Input: part model. Units: mm. Frame: model coordinates. Face numbers are marked on the shaded views. A direction names the side the tool comes from. Round coordinates to 2 decimals unless told otherwise and drop trailing zeros. Write each loop counter-clockwise with the first axis right and the second up, starting at its lowest first coordinate (ties: lowest second). Pieces come first, ordered by that corner, then holes. Notation, with made-up numbers: M 73,84 L 106,84 A4 ccw 106,89 Z; hole C -27.5,-4 d6. An arc over 180 degrees is marked long. Use one line per item in the form item = value. Start each with the question number.
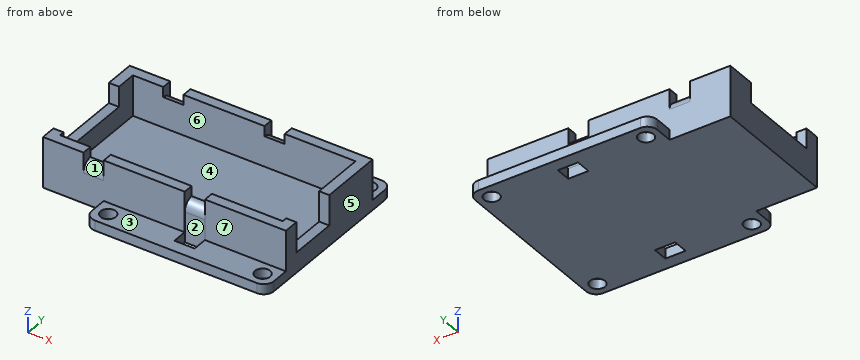
```python
from build123d import *

# Parameters (mm, degrees)
F1_DEPTH     = 2
F2_R         = 2
F3_D         = 3
F6_W         = 2
F6_H         = 9.5
F7_DEPTH     = 2
F6_W_2       = 4
F6_H_2       = 2
F6_H_3       = 1.9668334348
F8_DEPTH     = 8
F6_W_3       = 16
F9_DEPTH     = 10
F10_T1_DEPTH = 4
F10_T3_DEPTH = 4
F11_DEPTH    = 4
F6_H_4       = 16
F12_DEPTH    = 6


# Not quite as in the source:
# - a fillet or chamfer that OpenCascade refuses, or shapes differently, is made with other operations: its cross-section is extruded or revolved along the edge and cut away or added
# - a feature names something its author has since deleted; it is built from what else it names


with BuildPart() as f1:
    # F0 (on Top) → F1 (new body)
    with BuildSketch(Plane.XY):
        Polygon((-19.8978664808, -19.9668334348), (-1.8978664808, -19.9668334348), (-1.8978664808, -17.4668334348), (-3.8978664808, -17.4668334348), (-3.8978664808, -14.4668334348), (-1.8978664808, -14.4668334348), (-1.8978664808, -1.9668334348), (-19.8978664808, -1.9668334348), align=None)
    extrude(amount=F1_DEPTH)

    # F2
    f2_edges = [f1.edges().sort_by_distance(p)[0] for p in [
        (-19.897866, -19.966833, 1),
    ]]
    fillet(f2_edges, radius=F2_R)

    # F3 (through all)
    with Locations(Plane(origin=(0, 0, 0), x_dir=(1, 0, 0), z_dir=(0, 0, -1))):
        with Locations((-17.1478664808, 17.2168334348)):
            Hole(F3_D / 2)

    # F4: F1 across face


with BuildPart() as f1_1:
    add(f1.part)
    add(f1.part.mirror(Plane(origin=(-1.8978664808, -8.2168334348, 1), x_dir=(0, 1, 0), z_dir=(1, 0, 0))))

    # F5: F1 across face


with BuildPart() as f1_2:
    add(f1_1.part)
    add(f1_1.part.mirror(Plane(origin=(-1.8978664808, -1.9668334348, 1), x_dir=(-1, 0, 0), z_dir=(0, 1, 0))))

    # F6 (on face) → F7 (join)
    with BuildSketch(Plane(origin=(0, 0, 0), x_dir=(1, 0, 0), z_dir=(0, 0, -1))):
        Polygon((-29.8978664808, -8.5), (-23.8978664808, -8.5), (-19.8978664808, -8.5), (-19.8978664808, 12.5), (-23.8978664808, 12.5), (-29.8978664808, 12.5), (-29.8978664808, 11.5), (-29.8978664808, -4.5), align=None)
        with Locations((15.1021335192, 6.75)):
            Rectangle(F6_W, F6_H)
        Polygon((-19.8978664808, 12.5), (-19.8978664808, -8.5), (-3.8978664808, -8.5), (0.1021335192, -8.5), (14.1021335192, -8.5), (14.1021335192, 2), (14.1021335192, 11.5), (14.1021335192, 12.5), (0.1021335192, 12.5), (-3.8978664808, 12.5), align=None)
    extrude(amount=-F7_DEPTH)

    # F6 (on face) → F8 (join)
    with BuildSketch(Plane(origin=(0, 0, 0), x_dir=(1, 0, 0), z_dir=(0, 0, -1))):
        with Locations((-1.8978664808, -9.5)):
            Rectangle(F6_W_2, F6_H_2)
        with Locations((-1.8978664808, 13.4834167174)):
            Rectangle(F6_W_2, F6_H_3)
        with Locations((-21.8978664808, 13.5)):
            Rectangle(F6_W_2, F6_H_2)
        with Locations((-21.8978664808, -9.5)):
            Rectangle(F6_W_2, F6_H_2)
    extrude(amount=-F8_DEPTH)

    # F6 (on face) → F9 (join)
    with BuildSketch(Plane(origin=(0, 0, 0), x_dir=(1, 0, 0), z_dir=(0, 0, -1))):
        Polygon((-31.8978664808, -10.5), (-23.8978664808, -10.5), (-23.8978664808, -8.5), (-29.8978664808, -8.5), (-29.8978664808, -4.5), (-31.8978664808, -4.5), align=None)
        Polygon((0.1021335192, -8.5), (0.1021335192, -10.5), (16.1021335192, -10.5), (16.1021335192, 2), (14.1021335192, 2), (14.1021335192, -8.5), align=None)
        Polygon((0.1021335192, 14.4668334348), (0.1021335192, 12.5), (14.1021335192, 12.5), (14.1021335192, 11.5), (16.1021335192, 11.5), (16.1021335192, 14.5), (0.1021335192, 14.5), align=None)
        Polygon((-19.8978664808, 14.5), (-19.8978664808, 12.5), (-3.8978664808, 12.5), (-3.8978664808, 14.4668334348), (-3.8978664808, 14.5), align=None)
        Polygon((-31.8978664808, 14.5), (-31.8978664808, 11.5), (-29.8978664808, 11.5), (-29.8978664808, 12.5), (-23.8978664808, 12.5), (-23.8978664808, 14.5), align=None)
        with Locations((-11.8978664808, -9.5)):
            Rectangle(F6_W_3, F6_H_2)
    extrude(amount=-F9_DEPTH)

    # F10: fillet of radius 2 on 4 edges, made by hand

    # F10_s2 → F10_t1 (cut)
    with BuildSketch(Plane.YZ.offset(-3.8978664808)):
        with BuildLine():
            ThreePointArc((-14.4668334348, 6), (-13.8810469972, 7.4142135624), (-12.4668334348, 8))
            Line((-12.4668334348, 8), (-14.4668334348, 8))
            Line((-14.4668334348, 8), (-14.4668334348, 6))
        make_face()
        with BuildLine():
            ThreePointArc((8.5, 8), (9.9142135624, 7.4142135624), (10.5, 6))
            Line((10.5, 6), (10.5, 8))
            Line((10.5, 8), (8.5, 8))
        make_face()
    extrude(amount=F10_T1_DEPTH, mode=Mode.SUBTRACT)

    # F10_s4 → F10_t3 (cut)
    with BuildSketch(Plane.YZ.offset(-23.8978664808)):
        with BuildLine():
            ThreePointArc((8.5, 8), (9.9142135624, 7.4142135624), (10.5, 6))
            Line((10.5, 6), (10.5, 8))
            Line((10.5, 8), (8.5, 8))
        make_face()
        with BuildLine():
            ThreePointArc((-14.5, 6), (-13.9142135624, 7.4142135624), (-12.5, 8))
            Line((-12.5, 8), (-14.5, 8))
            Line((-14.5, 8), (-14.5, 6))
        make_face()
    extrude(amount=F10_T3_DEPTH, mode=Mode.SUBTRACT)

    # F6 (on face) → F11 (join)
    with BuildSketch(Plane(origin=(0, 0, 0), x_dir=(1, 0, 0), z_dir=(0, 0, -1))):
        with Locations((15.1021335192, 6.75)):
            Rectangle(F6_W, F6_H)
    extrude(amount=-F11_DEPTH)

    # F6 (on face) → F12 (join)
    with BuildSketch(Plane(origin=(0, 0, 0), x_dir=(1, 0, 0), z_dir=(0, 0, -1))):
        with Locations((-30.8978664808, 3.5)):
            Rectangle(F6_W, F6_H_4)
    extrude(amount=-F12_DEPTH)


solid = f1_2.part
```
Item 1: Cut plane B-B (x = -1). Give the number of separate pieces and of enclosed holes in the cut face, plus the area to 3 significant figures.
Item 2: First-contact query: pin 1 (4 mm diameter, centred on x = 8.5, z = 7.5, fed in from -Y); pin 2 (1.6 mm diameter, centred on y = 13, z = 0.5, fed in from -X); pin 3 (5 mm diameter, centred on x = -17.15, y = 13.28, fed in from -Z); pin 4 (1 mm diameter, centred on x = -17, z = 3.5, fed in from +Y). Flat tips, straight axial feed; report the tip coordinate or a pass-through.
Item 3: Draft query along Y for the marked faces 5, 6 and 7. Return one class per face: +Y half, -Y half, draft (parallel to the pull), parting line (faces both ways), or undercut.
Item 4: Reachability of the marked faces 1, 2, 3 and 4 from +Z, -Z, +X, -X, +Y, -Y: full face, straight path, thin tool, end or side. Return the list, or none.
Item 5: Ray query, line 1 (X direction, y = -14, z = 9.25); line 2 (Y direction, x = 6.5, z = 7); line 3 (X direction, y = 0, z = 2.75). Return the intervals inside material, ascending. Write a range as from..to.
Item 6: Cut plane D-D (y = -2.5). Output: boundary loops of the cut face in (x, z).
Final values:
q1.separate_pieces = 3
q1.enclosed_holes = 0
q1.area = 82.1 mm^2
q2.pin_1 = -14.5
q2.pin_2 = -19.9
q2.pin_3 = 0
q2.pin_4 = 10.5
q3.face_5 = draft
q3.face_6 = undercut
q3.face_7 = -Y half
q4.face_1 = +Z, -Y
q4.face_2 = +Z, -Z
q4.face_3 = +Z, +X, -X, -Y
q4.face_4 = +Z
q5.line_1 = -31.9..-23.9, -19.9..-3.9, 0.1..16.1
q5.line_2 = -14.5..-12.5, 8.5..10.5
q5.line_3 = -31.9..-29.9, 14.1..16.1
q6.outline = M -31.9,0 L 16.1,0 L 16.1,4 L 14.1,4 L 14.1,2 L -29.9,2 L -29.9,6 L -31.9,6 Z
